For this review, use the dimensioned drawing (mm, ordinates from the lowest corner) and the shaded views. Give positions to 0.01 mm unless a question says otherwise; leave off trailing zeros. Loops run counter-clockwise (first coordinate to the right, second up) from the corner with the lowest first, then second, coordinate; pieces in that order, holes last. Notation, with made-up numbers: M -15,7.5 L -9,7.5 A14 ccw -9,20.5 Z; hole C 21.25,-36 d7. An arc over 180 degrees is marked long. Use a Markdown table: item, result. Add a question column.
(1) Add section D-D, the plane x = 2. Give the boundary of the cut face in (y, z), then the cut area to 3 significant figures.
(2) Add section C-C, the plane x = 4. Give the boundary of the cut face in (y, z), then the cut area to 3 significant figures.
(3) Draft analysis for pull direction Z (two halves, no side actions). For the marked faces 1, 2 and 3, state which applies: pulls with the +Z half, pulls with the -Z half, needs draft (parallel to the pull), parting line crosses it, or undercut.
(4) Add section B-B, the plane y = 4.5. Give the boundary of the cut face in (x, z), then the cut area to 3 significant figures.
(5) Add section A-A, the plane z = 5. Give the boundary of the cut face in (x, y).
(6) For probe 1 along Y at (x, z) = (7, 3.25); probe 2 along Z at (x, y) = (8.25, 4.5) (3 decimals); probe 3 along Z at (x, y) = (2, 4.5), list the stretches that pass through material, from the lowest coordinate up.
(7) Insertion check: pin 1 Ø3 at (x, y) = (8, 1) entering from +Z; pin 2 Ø2 at (x, y) = (3.5, 8) entering from +Z; pin 3 Ø1 at (x, y) = (7, 4) entering from -Z. Each pin has a flat end and moves straight along its axis. Give the tip position at first contact, or say it passes through.
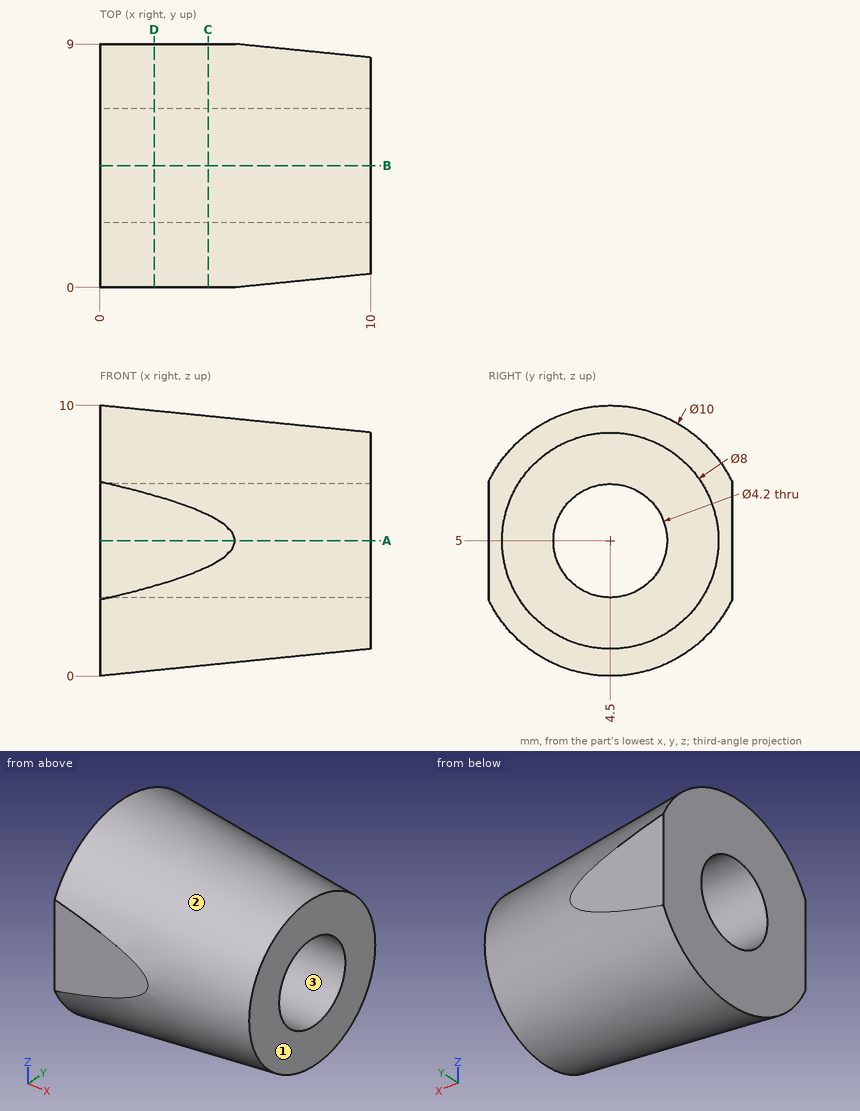
Established:
| question | item | result |
|---|---|---|
| 1 | outline | M 0,3.33 A4.8 ccw 9,3.33 L 9,6.67 A4.8 ccw 0,6.67 Z; hole C 4.5,5 d4.2 |
| 1 | area | 57.2 mm^2 |
| 2 | outline | M 0,4.05 A4.6 ccw 9,4.05 L 9,5.95 A4.6 ccw 0,5.95 Z; hole C 4.5,5 d4.2 |
| 2 | area | 52.4 mm^2 |
| 3 | face 1 | needs draft |
| 3 | face 2 | parting line crosses it |
| 3 | face 3 | undercut |
| 4 | outline | M 0,0 L 10,1 L 10,2.9 L 0,2.9 Z; M 0,7.1 L 10,7.1 L 10,9 L 0,10 Z |
| 4 | area | 48.0 mm^2 |
| 5 | outline | M 0,0 L 5,0 L 10,0.5 L 10,2.4 L 0,2.4 Z; M 0,6.6 L 10,6.6 L 10,8.5 L 5,9 L 0,9 Z |
| 6 | probe 1 | 0.57 to 3.34, 5.66 to 8.43 |
| 6 | probe 2 | 0.825 to 2.9, 7.1 to 9.175 |
| 6 | probe 3 | 0.2 to 2.9, 7.1 to 9.8 |
| 7 | pin 1 | z = 8.71 |
| 7 | pin 2 | z = 8.93 |
| 7 | pin 3 | z = 0.66 |
